from build123d import *

# Parameters (mm, degrees)
BOX_W             = 100
BOX_H             = 20
BOX_DEPTH         = 35
CYLINDER001_R     = 0.795
CYLINDER001_DEPTH = 15
FILLET_R          = 1


with BuildPart() as cube:
    # Box → Box (new body)
    with BuildSketch(Plane(origin=(500, -8.3245, -17.5), x_dir=(1, 0, 0), z_dir=(0, 0, 1))):
        with Locations((50, 10)):
            Rectangle(BOX_W, BOX_H)
    extrude(amount=BOX_DEPTH)


with BuildPart() as fillet_body:
    # Cylinder001 → Cylinder001 (new body)
    with BuildSketch(Plane(origin=(533.235, -7.5295, 0), x_dir=(1, 0, 0), z_dir=(0, -1, 0))):
        Circle(CYLINDER001_R)
    extrude(amount=CYLINDER001_DEPTH)

    # Fusion: union Cube
    add(cube.part)

    # Fillet
    fillet_edges = [fillet_body.edges().sort_by_distance(p)[0] for p in [
        (532.44, -8.3245, 0),
    ]]
    fillet(fillet_edges, radius=FILLET_R)


solid = fillet_body.part
Geometry: final body of the model. Coordinates: model frame, mm. Coordinates: 2 decimals unless noted, no trailing zeros. Loops run counter-clockwise (first coordinate to the right, second up) from the corner with the lowest first, then second, coordinate; pieces in that order, holes last. Notation, with made-up numbers: (-5, 19) - (4, 19) arc R13 ccw to (4, 29) - close; hole circle Ø7 at (-29, -30). An arc over 180 degrees is marked (long way). One line per question, with ' | ' between items. Start each with the question number.
(1) First-contact query: pin 1 (1 mm diameter, centred on x = 516.5, y = -9.5, fed in from -Z); pin 2 (2 mm diameter, centred on x = 549, z = -1.5, fed in from -Y). Flat tips, straight axial feed; report the tip coordinate or a pass-through.
(2) Draft query along Y for faces 1 (the flat face through (549, 11.676, 0)), 2 (the flat face through (549, -8.324, 0)), 3 (the flat face through (500, 2, 0)). Return one class per face: +Y half, -Y half, draft (parallel to the pull), parting line (faces both ways), or undercut.
(3) Ray query, L1, parallel to Y at x = 530, z = -10. Return the intervals inside material, ascending. Write a range as from..to.
(4) Cut plane A-A on x = 522. Output: boundary loops of the cut face in (y, z), and give its area (3 significant figures).
(5) Cut plane B-B on z = 14. Output: boundary loops of the cut face in (x, y), and give its area (3 significant figures).
Here are the results:
1) pin 1: through | pin 2: y = -8.32
2) face 1: +Y half | face 2: -Y half | face 3: draft
3) L1: -8.32..11.68
4) outline: (-8.32, -17.5) - (11.68, -17.5) - (11.68, 17.5) - (-8.32, 17.5) - close | area: 700 mm²
5) outline: (500, -8.32) - (600, -8.32) - (600, 11.68) - (500, 11.68) - close | area: 2,000 mm²
